Can you work these out from the model? Positions are in its coordinate system, mm. Face numbers are marked on the shaded views. A direction names the side the tool comes from. Coordinates: 2 decimals unless noted, no trailing zeros. Loops run counter-clockwise (first coordinate to the right, second up) from the corner with the lowest first, then second, coordinate; pieces in that order, holes last.
Autodesk Inventor part; units mm, degrees
ref_plane "РабПлоскость1" through (0, 0, 39.2) normal (0, 0, 1) x (1, 0, 0)
ref_plane "YZ Plane" through (0, 0, 0) normal (1, 0, 0) x (0, 1, 0)
ref_plane "XZ Plane" through (0, 0, 0) normal (0, 1, 0) x (-1, 0, 0)
ref_plane "РабПлоскость1" through (0, 0, 39.2) normal (0, 0, 1) x (1, 0, 0)
sketch "Эскиз1" plane through (0, 0, 39.2) normal (0, 0, 1) x (1, 0, 0)
  line L0 (27.5, -32.5) -> (-27.5, -32.5)
  line L1 (-32.5, -27.5) -> (-32.5, 27.5)
  line L2 (-27.5, 32.5) -> (27.5, 32.5)
  line L3 (32.5, 27.5) -> (32.5, -27.5)
  line L4 (32.5, -32.5) -> (-32.5, 32.5) construction
  line L5 (-32.5, -32.5) -> (32.5, 32.5) construction
  circle A0 centre (-15.35, 15.35) radius 1.75 construction
  circle A1 centre (15.35, 15.35) radius 1.75 construction
  arc A2 (14.0855, -15.35) -> (14.4559, -14.4559) centre (15.35, -15.35) ccw construction
  arc A3 (-16.6145, -15.35) -> (-16.2441, -14.4559) centre (-15.35, -15.35) ccw construction
  line L6 (-27.5, 32.5) -> (-32.5, 27.5)
  line L7 (-32.5, -27.5) -> (-27.5, -32.5)
  line L8 (27.5, -32.5) -> (32.5, -27.5)
  line L9 (27.5, 32.5) -> (32.5, 27.5)
  circle A4 centre (0, 0) radius 10.7 construction
  circle A5 centre (0, 0) radius 8.46 construction
  circle A6 centre (0, 0) radius 11.5
  dimension "d0" = 65
  dimension "d1" = 5
  dimension "d2" = 5
  dimension "d3" = 5
  dimension "d4" = 5
  dimension "d5" = 5
  dimension "d6" = 5
  dimension "d7" = 5
  dimension "d8" = 5
  dimension "d9" = 23
extrude "Выдавливание1" add sketch "Эскиз1" along normal blind 4
sketch "Эскиз2" plane through (0, 0, 43.2) normal (0, 0, 1) x (1, 0, 0)
  line L0 (15.35, -15.35) -> (-15.35, -15.35) construction
  line L1 (-15.35, -15.35) -> (-15.35, 15.35) construction
  line L2 (-15.35, 15.35) -> (15.35, 15.35) construction
  line L3 (15.35, 15.35) -> (15.35, -15.35) construction
  line L4 (15.35, -15.35) -> (-15.35, 15.35) construction
  line L5 (-15.35, -15.35) -> (15.35, 15.35) construction
  point P0 (0, 0)
  dimension "d12" = 30.7
hole "Отверстие1" at (-15.35, 15.35, 43.2) at (15.35, 15.35, 43.2) at (15.35, -15.35, 43.2) at (-15.35, -15.35, 43.2) direction (0, 0, -1) diameter 3.4 end through all countersink diameter 6.6 countersink angle 90
sketch "Эскиз3" plane through (0, 0, 43.2) normal (0, 0, 1) x (1, 0, 0)
  line L0 (26.4645, -26.4645) -> (-26.4645, -26.4645) construction
  line L1 (-26.4645, -26.4645) -> (-26.4645, 26.4645) construction
  line L2 (-26.4645, 26.4645) -> (26.4645, 26.4645) construction
  line L3 (26.4645, 26.4645) -> (26.4645, -26.4645) construction
  line L4 (26.4645, -26.4645) -> (-26.4645, 26.4645) construction
  line L5 (-26.4645, -26.4645) -> (26.4645, 26.4645) construction
  line L6 (-27.5, 32.5) -> (-32.5, 27.5) construction
  point P0 (0, 0)
  point P1 (-30, 30)
  dimension "d31" = 5
hole "Отверстие2" at (-26.4645, 26.4645, 43.2) at (26.4645, 26.4645, 43.2) at (26.4645, -26.4645, 43.2) at (-26.4645, -26.4645, 43.2) direction (0, 0, -1) diameter 3.9 end through all
sketch "Эскиз4" plane through (0, 0, 43.2) normal (0, 0, 1) x (1, 0, 0)
  circle A0 centre (0, 0) radius 12.5
  circle A1 centre (0, 0) radius 11.5
  dimension "d28" = 1
extrude "Выдавливание2" add sketch "Эскиз4" along normal blind 1
chamfer "Фаска1" distance 1.4 angle 45 4 edges at (-26.4645, -24.5145, 39.2) (26.4645, -24.5145, 39.2) (-26.4645, 28.4145, 39.2) (26.4645, 28.4145, 39.2)
equation "\"d2\" = d1"
equation "\"d3\" = d1"
equation "\"d4\" = d3"
equation "\"d5\" = d1"
equation "\"d6\" = d5"
equation "\"d7\" = d1"
equation "\"d8\" = d7"
properties part number "Основание_нижнее" material "По умолчанию1"
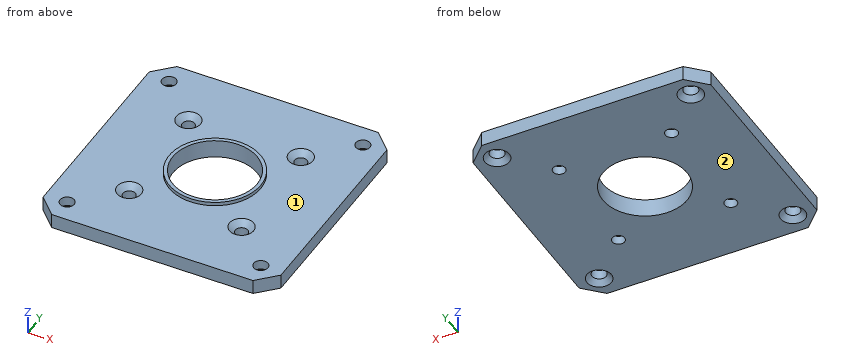
(1) I want a section at B-B on y = 0. Write out the boundary of the cut face in (x, z), then the cut area to 3 significant figures.
Check values:
outline: (-32.5, 39.2) - (-11.5, 39.2) - (-11.5, 44.2) - (-12.5, 44.2) - (-12.5, 43.2) - (-32.5, 43.2) - close; (11.5, 39.2) - (32.5, 39.2) - (32.5, 43.2) - (12.5, 43.2) - (12.5, 44.2) - (11.5, 44.2) - close
area: 170 mm2
(2) Which directions (+Z, -Z, +X, -X, +Y, -Y) give clear straight access to the entire face, cutting with the end or side of a thin tool? Please do the marked faces 1 and 2.
Check values:
face 1: +Z
face 2: -Z, +X, -X, +Y, -Y
(3) I'm going to push flat-ended pins straight in: pin 1 (6 mm diameter, centred on x = -26.46, y = 26.46, fed in from +Z); pin 2 (6 mm diameter, centred on x = 26.46, y = 26.46, fed in from -Z); pin 3 (6 mm diameter, centred on x = 8.5, y = -5.5, fed in from +Z); pin 4 (4.5 mm diameter, centred on x = 15.35, y = 15.35, fed in from +Z). Where does each tip first touch, or does it pass through?
Check values:
pin 1: stops at z = 43.2
pin 2: stops at z = 39.54
pin 3: stops at z = 44.2
pin 4: stops at z = 42.15
(4) I want a section at D-D on x = -0.5. Write out the boundary of the cut face in (y, z), then the cut area to 3 significant figures.
Check values:
outline: (-32.5, 39.2) - (-11.49, 39.2) - (-11.49, 44.2) - (-12.49, 44.2) - (-12.49, 43.2) - (-32.5, 43.2) - close; (11.49, 39.2) - (32.5, 39.2) - (32.5, 43.2) - (12.49, 43.2) - (12.49, 44.2) - (11.49, 44.2) - close
area: 170 mm2
(5) I want a section at A-A on x = -15.35. Write out the boundary of the cut face in (y, z).
Check values:
outline: (-32.5, 39.2) - (-17.05, 39.2) - (-17.05, 41.6) - (-18.65, 43.2) - (-32.5, 43.2) - close; (-13.65, 39.2) - (13.65, 39.2) - (13.65, 41.6) - (12.05, 43.2) - (-12.05, 43.2) - (-13.65, 41.6) - close; (17.05, 39.2) - (32.5, 39.2) - (32.5, 43.2) - (18.65, 43.2) - (17.05, 41.6) - close
(6) If I drill on probe 1 along Y at (x, z) = (-15.35, 40.75); probe 2 along X at (y, z) = (-14.5, 43.15), over which ranges is the centre line in solid material (lowest first)?
Check values:
probe 1: y = -32.5 to -17.05, -13.65 to 13.65, 17.05 to 32.5
probe 2: x = -32.5 to -18.49, -12.21 to 12.21, 18.49 to 32.5
